```python
from build123d import *

# Parameters (mm, degrees)
F1_DEPTH = 19.05
F3_DEPTH = 6.35
F4_R     = 2.1395052033
F4_R_2   = 1.5473789097
F4_W     = 4.3834099779
F4_H     = 1.2019015849
F5_DEPTH = 0.635


with BuildPart() as f1:
    # F0 (on Front) → F1 (new body)
    with BuildSketch(Plane.XZ):
        Polygon((12.7812118899, 24.9824322697), (0, 75.4986554384), (-12.7812118899, 24.9824322697), (-17.9893098468, 4.3980431727), (17.9893098468, 4.3980431727), align=None)
        with BuildLine():
            Line((17.9893098468, 4.3980431727), (-17.9893098468, 4.3980431727))
            Line((-17.9893098468, 4.3980431727), (-44.1846288741, -12.0744779706))
            Line((-44.1846288741, -12.0744779706), (-39.6815885197, -14.3474328787))
            Line((-39.6815885197, -14.3474328787), (-41.1387868226, -19.7073649615))
            ThreePointArc((-41.1387868226, -19.7073649615), (-38.4139838362, -23.6659590485), (-33.6108808251, -23.5071512254))
            Line((-33.6108808251, -23.5071512254), (-32.1536825222, -18.1472191426))
            Line((-32.1536825222, -18.1472191426), (-24.6516230519, -21.933959112))
            Line((-24.6516230519, -21.933959112), (-29.4550578464, -40.9189650839))
            Line((-29.4550578464, -40.9189650839), (-8.3569039417, -38.1258840272))
            Line((-8.3569039417, -38.1258840272), (-8.3569039417, -46.5887725028))
            add(Edge.make_bspline(
                [(-8.3569039417, -46.5887725028), (-7.1639467181, -46.4381227358), (-6.0970060344, -46.567074298), (-5.1892242436, -47.0491623459)],
                knots=[0.3623606656, 0.3623606656, 0.3623606656, 0.3623606656, 0.4576615295, 0.4576615295, 0.4576615295, 0.4576615295], degree=3))
            Line((-5.1892242436, -47.0491623459), (-5.1892242436, -37.7065304572))
            Line((-5.1892242436, -37.7065304572), (0, -37.0195545256))
            Line((0, -37.0195545256), (5.1886305738, -37.7110000757))
            Line((5.1886305738, -37.7110000757), (5.1805830548, -47.0536284984))
            add(Edge.make_bspline(
                [(8.3486581466, -46.5959673895), (7.1558311316, -46.4442900935), (6.0887797679, -46.5723225708), (5.1805830548, -47.0536284984)],
                knots=[0.3623606656, 0.3623606656, 0.3623606656, 0.3623606656, 0.4576615295, 0.4576615295, 0.4576615295, 0.4576615295], degree=3))
            Line((8.3486581466, -46.5959673895), (8.3559478758, -38.1330820534))
            Line((8.3559478758, -38.1330820534), (29.4550578464, -40.9189650839))
            Line((29.4550578464, -40.9189650839), (24.6516230519, -21.933959112))
            Line((24.6516230519, -21.933959112), (32.1536825222, -18.1472191426))
            Line((32.1536825222, -18.1472191426), (33.6108808251, -23.5071512254))
            ThreePointArc((33.6108808251, -23.5071512254), (38.4139838362, -23.6659590485), (41.1387868226, -19.7073649615))
            Line((41.1387868226, -19.7073649615), (39.6815885197, -14.3474328787))
            Line((39.6815885197, -14.3474328787), (44.1846288741, -12.0744779706))
            Line((44.1846288741, -12.0744779706), (17.9893098468, 4.3980431727))
        make_face()
        with BuildLine():
            add(Edge.make_bspline(
                [(-8.3569039417, -46.5887725028), (-7.1639467181, -46.4381227358), (-6.0970060344, -46.567074298), (-5.1892242436, -47.0491623459)],
                knots=[0.3623606656, 0.3623606656, 0.3623606656, 0.3623606656, 0.4576615295, 0.4576615295, 0.4576615295, 0.4576615295], degree=3))
            add(Edge.make_bspline(
                [(-25.6085079163, -56.3917942345), (-19.2506852316, -51.7766897434), (-12.8928625468, -47.1615852522), (-8.3569039417, -46.5887725028)],
                knots=[0, 0, 0, 0, 0.3623606656, 0.3623606656, 0.3623606656, 0.3623606656], degree=3))
            Line((-25.6085079163, -56.3917942345), (-18.7088064849, -56.3917942345))
            Line((-18.7088064849, -56.3917942345), (-10.747612454, -51.8804490566))
            Line((-10.747612454, -51.8804490566), (-10.747612454, -56.3917942345))
            Line((-10.747612454, -56.3917942345), (-5.1892242436, -56.3917942345))
            Line((-5.1892242436, -56.3917942345), (-5.1892242436, -47.0491623459))
        make_face()
        with BuildLine():
            add(Edge.make_bspline(
                [(25.5918116332, -56.4138456024), (19.2379666475, -51.7932663474), (12.8841216618, -47.1726870923), (8.3486581466, -46.5959673895)],
                knots=[0, 0, 0, 0, 0.3623606656, 0.3623606656, 0.3623606656, 0.3623606656], degree=3))
            add(Edge.make_bspline(
                [(8.3486581466, -46.5959673895), (7.1558311316, -46.4442900935), (6.0887797679, -46.5723225708), (5.1805830548, -47.0536284984)],
                knots=[0.3623606656, 0.3623606656, 0.3623606656, 0.3623606656, 0.4576615295, 0.4576615295, 0.4576615295, 0.4576615295], degree=3))
            Line((5.1805830548, -47.0536284984), (5.1725355357, -56.396256921))
            Line((5.1725355357, -56.396256921), (10.730921684, -56.4010447834))
            Line((10.730921684, -56.4010447834), (10.7348076486, -51.8897012791))
            Line((10.7348076486, -51.8897012791), (18.6921127615, -56.407902365))
            Line((18.6921127615, -56.407902365), (25.5918116332, -56.4138456024))
        make_face()
    extrude(amount=F1_DEPTH)

    # F2 (on face) → F3 (join)
    with BuildSketch(Plane.XZ.offset(19.05)):
        Polygon((12.7791271915, 24.9906717928), (0, 48.4305992723), (-12.7791271915, 24.9906717928), (0, 7.8285075724), align=None)
    extrude(amount=F3_DEPTH)

    # F4 (on face) → F5 (join)
    with BuildSketch(Plane.XZ.offset(25.4)):
        with Locations((-3.0517904088, 30.9159699827)):
            Circle(F4_R)
        with Locations((2.2556707263, 30.6505970657)):
            Circle(F4_R_2)
        Polygon((5.0654464612, 18.4789821506), (-3.9945594035, 18.4789821506), (-3.6306733055, 17.9902889184), (4.7015603632, 17.9902889184), align=None)
        with Locations((-3.4289575997, 35.0581686944)):
            Rectangle(F4_W, F4_H)
        with Locations((3.4996584873, 35.0581686944)):
            Rectangle(F4_W, F4_H)
    extrude(amount=F5_DEPTH)


solid = f1.part
```
Design review of the part built by this model. Coordinates are the model's own, in mm. A direction names the side the tool comes from. Coordinates: 2 decimals unless noted, no trailing zeros. Write each loop counter-clockwise with the first axis right and the second up, starting at its lowest first coordinate (ties: lowest second). Pieces come first, ordered by that corner, then holes.
1) Add section C-C (y = -21.5). Write out the cut boundary in (x, z).
2) Insertion check: pin 1 (6 mm diameter, centred on y = -10, z = 9, fed in from -X); pin 2 (7 mm diameter, centred on y = -8, z = -41, fed in from -X); pin 3 (10 mm diameter, centred on x = -32, y = -11.5, fed in from +Z); pin 4 (4 mm diameter, centred on x = -10.5, z = 9, fed in from +Y). Each pin has a flat end and moves straight along its axis. Give the tip position at first contact, or say it passes through.
3) Machinability: for faces 1 (the flat face through (-41.965, -9.392, -13.195)), 2 (the flat face through (6.3, -22.18, 16.29)), 3 (the flat face through (-1, -19.05, 48)), 4 (the flat face through (-5.189, -9, -47)), which of the approach directions +Z, -Z, +X, -X, +Y, -Y give a long, thin tool a straight path to every point of the face, cutting with its end or side? Answer none if there is none.
4) To check wall thickness, follow L1, parallel to Y at x = -10, z = -37.5; L2, parallel to X at y = -17.75, z = -44.5; L3, parallel to Y at x = -8, z = 25. State the ranges of each line that lie inside material, in increasing order.
5) Mouldability with a two-part tool opening along X and no side actions: class faces 5 (the flat face through (-6.48, -22.18, 16.53)), 6 (the flat face through (31.27, -9.392, -3.954)), 7 (the flat face through (14.66, -9.39, -54.12)), 8 (the flat face through (-8, -9, -56.392)) as +X half, -X half, draft (parallel to the pull), parting line (faces both ways), or undercut.
6) Add section D-D (z = 20.5). Write out the cut boundary in (x, y).
7) Add section B-B (z = 45). Write out the cut boundary in (x, y).
8) Add section A-A (x = -27). Write out the cut boundary in (y, z).
Check result:
1. outline: (-12.78, 24.99) - (0, 7.83) - (12.78, 24.99) - (0, 48.43) - close
2. pin 1: stops at x = -17.58
2. pin 2: stops at x = -29.46
2. pin 3: stops at z = -1.27
2. pin 4: stops at y = 0
3. face 1: -X, +Y, -Y
3. face 2: -Z, +X, -Y
3. face 3: +Z, -Y
3. face 4: -Z, +Y, -Y
4. L1: y = -19.05 to 0
4. L2: x = -8.36 to -5.19, 5.18 to 8.35
4. L3: y = -25.4 to 0
5. face 5: -X half
5. face 6: +X half
5. face 7: undercut
5. face 8: draft
6. outline: (-13.92, -19.05) - (-9.44, -19.05) - (-9.44, -25.4) - (9.44, -25.4) - (9.44, -19.05) - (13.92, -19.05) - (13.92, 0) - (-13.92, 0) - close
7. outline: (-7.72, -19.05) - (-1.87, -19.05) - (-1.87, -25.4) - (1.87, -25.4) - (1.87, -19.05) - (7.72, -19.05) - (7.72, 0) - (-7.72, 0) - close
8. outline: (-19.05, -40.59) - (0, -40.59) - (0, -31.22) - (-19.05, -31.22) - close; (-19.05, -20.75) - (0, -20.75) - (0, -1.27) - (-19.05, -1.27) - close
